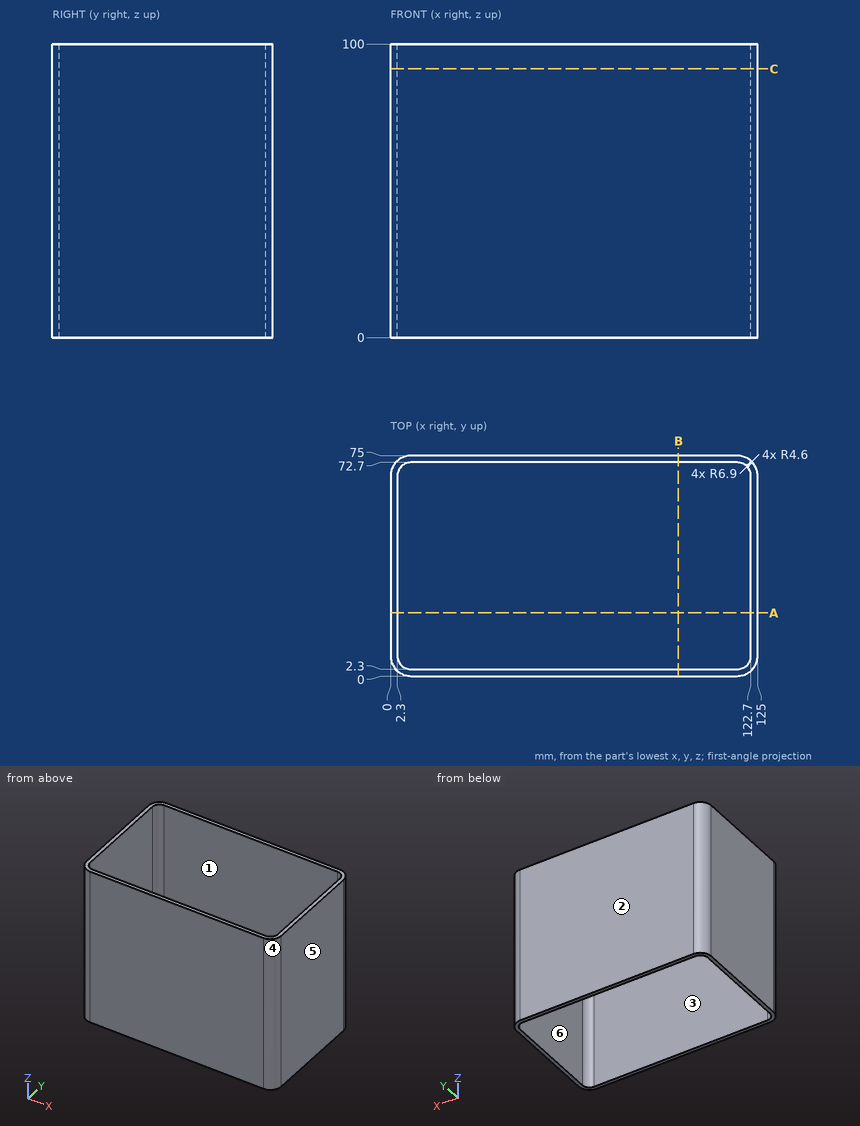
Could you check a few things on this drawing? It's one solid part, dimensions in mm from its lowest x, y, z. A direction names the side the tool comes from. Give positions to 0.01 mm unless a question says otherwise; leave off trailing zeros. Order: outer loops, then holes, each group sorted by start corner. A loop starts at its lowest first (then second) coordinate and runs counter-clockwise, first axis right, second up. Notation, with made-up numbers: M 16,-34 L 74,-34 A20 cw 74,-5 Z; hole C 88.25,-23.75 d10. An arc over 180 degrees is marked long. Use one line per item in the form item = value. Start each with the question number.
Item 1: We'd pull the mould along Y, two halves only. Please class the marked faces 1, 2, 3 and 4: +Y half, -Y half, draft (parallel to the pull), parting line (faces both ways), or undercut.
Item 2: For the marked faces 5 and 6, which set-ups out of +Z, -Z, +X, -X, +Y, -Y let a thin tool reach every point of the face, with its end or its side?
Item 3: If we section it at B-B (x = 98): Write out the boundary of the cut face in (y, z).
Item 4: If we section it at A-A (y = 21.5): Write out the boundary of the cut face in (x, z), then the cut area to 3 significant figures.
Item 5: If I drill on line 1 along Y through (x, z) = (39.5, 71); line 2 along X through (y, z) = (48, 30); line 3 along X through (y, z) = (4, 70), over which ranges is the centre line in solid material (lowest first)?
Item 6: If we section it at C-C (z = 91.5): Write out the boundary of the cut face in (x, y).
Outcome:
q1.face_1 = undercut
q1.face_2 = +Y half
q1.face_3 = undercut
q1.face_4 = -Y half
q2.face_5 = +Z, -Z, +X, +Y, -Y
q2.face_6 = +Z, -Z
q3.outline = M 0,0 L 2.3,0 L 2.3,100 L 0,100 Z; M 72.7,0 L 75,0 L 75,100 L 72.7,100 Z
q4.outline = M 0,0 L 2.3,0 L 2.3,100 L 0,100 Z; M 122.7,0 L 125,0 L 125,100 L 122.7,100 Z
q4.area = 460 mm2
q5.line_1 = 0 to 2.3, 72.7 to 75
q5.line_2 = 0 to 2.3, 122.7 to 125
q5.line_3 = 0.64 to 3.33, 121.67 to 124.36
q6.outline = M 0,6.9 A6.9 ccw 6.9,0 L 118.1,0 A6.9 ccw 125,6.9 L 125,68.1 A6.9 ccw 118.1,75 L 6.9,75 A6.9 ccw 0,68.1 Z; hole M 2.3,6.9 A4.6 ccw 6.9,2.3 L 118.1,2.3 A4.6 ccw 122.7,6.9 L 122.7,68.1 A4.6 ccw 118.1,72.7 L 6.9,72.7 A4.6 ccw 2.3,68.1 Z
